Build history of the part. All positions in model axes, mm. A direction names the side the tool comes from. Give positions to 0.01 mm unless a question says otherwise; leave off trailing zeros. Write each loop counter-clockwise with the first axis right and the second up, starting at its lowest first coordinate (ties: lowest second). Pieces come first, ordered by that corner, then holes. Notation, with made-up numbers: M -1,50 L 44,50 A22 cw 44,70 Z; hole C 47.25,-26.75 d9. An arc over 180 degrees is marked long. One line per item, written item: value. Start each with the question number.
from build123d import *

# Parameters (mm, degrees)
SKETCH_1_R           = 1.6
EXTRUDE_1_DEPTH      = 2
SKETCH_2_R           = 12.5
CUT_EXTRUDE_1_DEPTH  = 3
SKETCH_5_R           = 26
SKETCH_5_R_2         = 22
EXTRUDE_3_DEPTH      = 10
EXTRUDE_5_DEPTH      = 10
SKETCH_15_R          = 1.65
CUT_EXTRUDE_2_DEPTH  = 42
SKETCH_16_R          = 1.65
CUT_EXTRUDE_3_DEPTH  = 42
CUT_EXTRUDE_4_DEPTH  = 18
CUT_EXTRUDE_5_DEPTH  = 18
EXTRUDE_6_DEPTH      = 45
SKETCH_24_W          = 50.26
SKETCH_24_H          = 14
EXTRUDE_7_DEPTH      = 5
SKETCH_25_R          = 1.65
CUT_EXTRUDE_6_DEPTH  = 5
CUT_EXTRUDE_7_DEPTH  = 3
CUT_EXTRUDE_9_DEPTH  = 10
CUT_EXTRUDE_START    = -8
CUT_EXTRUDE_10_DEPTH = 8
SKETCH_34_W          = 26
SKETCH_34_H          = 14
EXTRUDE_9_DEPTH      = 5
SKETCH_35_R          = 1.65
CUT_EXTRUDE_11_DEPTH = 5
CUT_EXTRUDE_12_DEPTH = 3
SKETCH_37_W          = 3
SKETCH_37_H          = 14
EXTRUDE_10_DEPTH     = 14


with BuildPart() as part:
    # 草图1 → 凸台-拉伸1 (new body)
    with BuildSketch(Plane(origin=(0, 0, 0), x_dir=(1, 0, 0), z_dir=(0, 1, 0))):
        with BuildLine():
            ThreePointArc((20.341082498, 8.380952381), (0, 22), (-20.341082498, 8.380952381))
            ThreePointArc((-20.341082498, 8.380952381), (-4.271778613, -21.581286048), (22, 0))
            ThreePointArc((22, 0), (21.581286048, 4.271778613), (20.341082498, 8.380952381))
        make_face()
        with Locations(Location((-12.727922061, -12.727922061, 0), (0, 0, 270))):
            Circle(SKETCH_1_R, mode=Mode.SUBTRACT)
        with Locations(Location((12.727922061, -12.727922061, 0), (0, 0, 270))):
            Circle(SKETCH_1_R, mode=Mode.SUBTRACT)
        with Locations(Location((-12.727922061, 12.727922061, 0), (0, 0, 270))):
            Circle(SKETCH_1_R, mode=Mode.SUBTRACT)
        with Locations(Location((12.727922061, 12.727922061, 0), (0, 0, 270))):
            Circle(SKETCH_1_R, mode=Mode.SUBTRACT)
    extrude(amount=EXTRUDE_1_DEPTH)

    # 草图2 → 切除-拉伸1 (cut)
    with BuildSketch(Plane(origin=(0, 2, 0), x_dir=(1, 0, 0), z_dir=(0, 1, 0))):
        with Locations(Location((0, 0, 0), (0, 0, 270))):
            Circle(SKETCH_2_R)
    extrude(amount=-CUT_EXTRUDE_1_DEPTH, mode=Mode.SUBTRACT)

    # 草图5 → 凸台-拉伸3 (add)
    with BuildSketch(Plane(origin=(0, 0, 0), x_dir=(1, 0, 0), z_dir=(0, 1, 0))):
        with Locations(Location((0, 0, 0), (0, 0, 270))):
            Circle(SKETCH_5_R)
        with Locations(Location((0, 0, 0), (0, 0, 270))):
            Circle(SKETCH_5_R_2, mode=Mode.SUBTRACT)
    extrude(amount=EXTRUDE_3_DEPTH)

    # 草图14 → 凸台-拉伸5 (add)
    with BuildSketch(Plane.XZ):
        with BuildLine():
            Line((-10.307764064, 20), (10.307764064, 20))
            ThreePointArc((10.307764064, 20), (15.909902577, 15.909902577), (20, 10.307764064))
            Line((20, 10.307764064), (20, -10.307764064))
            ThreePointArc((20, -10.307764064), (15.909902577, -15.909902577), (10.307764064, -20))
            Line((10.307764064, -20), (-10.307764064, -20))
            ThreePointArc((-10.307764064, -20), (-15.909902577, -15.909902577), (-20, -10.307764064))
            Line((-20, -10.307764064), (-20, 10.307764064))
            ThreePointArc((-20, 10.307764064), (-15.909902577, 15.909902577), (-10.307764064, 20))
        make_face()
        with BuildLine():
            Line((-9.013878189, 15), (9.013878189, 15))
            ThreePointArc((9.013878189, 15), (9.692559275, 14.570665555), (10.350828667, 14.110646544))
            ThreePointArc((10.350828667, 14.110646544), (14.67246571, 14.67246571), (14.110646544, 10.350828667))
            ThreePointArc((14.110646544, 10.350828667), (14.570665555, 9.692559275), (15, 9.013878189))
            Line((15, 9.013878189), (15, -9.013878189))
            ThreePointArc((15, -9.013878189), (14.570665555, -9.692559275), (14.110646544, -10.350828667))
            ThreePointArc((14.110646544, -10.350828667), (14.67246571, -14.67246571), (10.350828667, -14.110646544))
            ThreePointArc((10.350828667, -14.110646544), (9.692559275, -14.570665555), (9.013878189, -15))
            Line((9.013878189, -15), (-9.013878189, -15))
            ThreePointArc((-9.013878189, -15), (-9.692559275, -14.570665555), (-10.350828667, -14.110646544))
            ThreePointArc((-10.350828667, -14.110646544), (-14.67246571, -14.67246571), (-14.110646544, -10.350828667))
            ThreePointArc((-14.110646544, -10.350828667), (-14.570665555, -9.692559275), (-15, -9.013878189))
            Line((-15, -9.013878189), (-15, 9.013878189))
            ThreePointArc((-15, 9.013878189), (-14.570665555, 9.692559275), (-14.110646544, 10.350828667))
            ThreePointArc((-14.110646544, 10.350828667), (-14.67246571, 14.67246571), (-10.350828667, 14.110646544))
            ThreePointArc((-10.350828667, 14.110646544), (-9.692559275, 14.570665555), (-9.013878189, 15))
        make_face(mode=Mode.SUBTRACT)
    extrude(amount=EXTRUDE_5_DEPTH)

    # 草图15 → 切除-拉伸2 (cut)
    with BuildSketch(Plane.ZY.offset(20)):
        with Locations((0, -5)):
            Circle(SKETCH_15_R)
    extrude(amount=-CUT_EXTRUDE_2_DEPTH, mode=Mode.SUBTRACT)

    # 草图16 → 切除-拉伸3 (cut)
    with BuildSketch(Plane(origin=(0, 0, -20), x_dir=(-1, 0, 0), z_dir=(0, 0, -1))):
        with Locations((0, -5)):
            Circle(SKETCH_16_R)
    extrude(amount=-CUT_EXTRUDE_3_DEPTH, mode=Mode.SUBTRACT)

    # 草图18 → 切除-拉伸4 (cut, symmetric)
    with BuildSketch(Plane.XY):
        Polygon((-1.58771324, -2.25), (-3.175426481, -5), (-1.58771324, -7.75), (1.58771324, -7.75), (3.175426481, -5), (1.58771324, -2.25), align=None)
    extrude(amount=CUT_EXTRUDE_4_DEPTH, both=True, mode=Mode.SUBTRACT)

    # 草图19 → 切除-拉伸5 (cut, symmetric)
    with BuildSketch(Plane(origin=(0, 0, 0), x_dir=(0, 0, -1), z_dir=(1, 0, 0))):
        Polygon((-1.58771324, -2.25), (-3.175426481, -5), (-1.58771324, -7.75), (1.58771324, -7.75), (3.175426481, -5), (1.58771324, -2.25), align=None)
    extrude(amount=CUT_EXTRUDE_5_DEPTH, both=True, mode=Mode.SUBTRACT)

    # 草图23 → 凸台-拉伸6 (add)
    with BuildSketch(Plane(origin=(0, 10, 0), x_dir=(1, 0, 0), z_dir=(0, 1, 0))):
        with BuildLine():
            ThreePointArc((-22, 0), (-21.712282003, 3.546379878), (-20.856653615, 7))
            Line((-20.856653615, 7), (-25.039968051, 7))
            ThreePointArc((-25.039968051, 7), (-25.758873901, 3.53276313), (-26, 0))
            Line((-26, 0), (-22, 0))
        make_face()
        with BuildLine():
            ThreePointArc((-20.856653615, -7), (-21.712282003, -3.546379878), (-22, 0))
            Line((-22, 0), (-26, 0))
            ThreePointArc((-26, 0), (-25.758873901, -3.53276313), (-25.039968051, -7))
            Line((-25.039968051, -7), (-20.856653615, -7))
        make_face()
        with BuildLine():
            Line((25.039968051, 7), (20.856653615, 7))
            ThreePointArc((20.856653615, 7), (21.712282003, 3.546379878), (22, 0))
            Line((22, 0), (26, 0))
            ThreePointArc((26, 0), (25.758873901, 3.53276313), (25.039968051, 7))
        make_face()
        with BuildLine():
            Line((26, 0), (22, 0))
            ThreePointArc((22, 0), (21.712282003, -3.546379878), (20.856653615, -7))
            Line((20.856653615, -7), (25.039968051, -7))
            ThreePointArc((25.039968051, -7), (25.758873901, -3.53276313), (26, 0))
        make_face()
    extrude(amount=EXTRUDE_6_DEPTH)

    # 草图24 → 凸台-拉伸7 (add)
    with BuildSketch(Plane(origin=(0, 55, 0), x_dir=(1, 0, 0), z_dir=(0, 1, 0))):
        with Locations((-50.169968051, 0)):
            Rectangle(SKETCH_24_W, SKETCH_24_H)
    extrude_7 = extrude(amount=-EXTRUDE_7_DEPTH)

    # 镜向1: 凸台-拉伸7 across plane
    add(extrude_7.mirror(Plane(origin=(0, 0, 0), x_dir=(0, 0, 1), z_dir=(1, 0, 0))))

    # 草图25 → 切除-拉伸6 (cut)
    with BuildSketch(Plane(origin=(0, 55, 0), x_dir=(1, 0, 0), z_dir=(0, 1, 0))):
        with Locations(Location((-60.299968051, 0, 0), (0, 0, 270))):
            Circle(SKETCH_25_R)
        with Locations(Location((-30.299968051, 0, 0), (0, 0, 270))):
            Circle(SKETCH_25_R)
    cut_extrude_6 = extrude(amount=-CUT_EXTRUDE_6_DEPTH, mode=Mode.SUBTRACT)

    # 草图26 → 切除-拉伸7 (cut)
    with BuildSketch(Plane(origin=(0, 50, 0), x_dir=(1, 0, 0), z_dir=(0, 1, 0))):
        Polygon((-58.712254811, 2.75), (-61.887681291, 2.75), (-63.475394532, 0), (-61.887681291, -2.75), (-58.712254811, -2.75), (-57.124541571, 0), align=None)
        Polygon((-31.887681291, 2.75), (-33.475394532, 0), (-31.887681291, -2.75), (-28.712254811, -2.75), (-27.124541571, 0), (-28.712254811, 2.75), align=None)
    cut_extrude_7 = extrude(amount=CUT_EXTRUDE_7_DEPTH, mode=Mode.SUBTRACT)

    # 镜向3: 切除-拉伸6, 切除-拉伸7 across plane
    add(cut_extrude_6.mirror(Plane(origin=(0, 0, 0), x_dir=(0, 0, 1), z_dir=(1, 0, 0))), mode=Mode.SUBTRACT)
    add(cut_extrude_7.mirror(Plane(origin=(0, 0, 0), x_dir=(0, 0, 1), z_dir=(1, 0, 0))), mode=Mode.SUBTRACT)

    # 草图28 → 切除-拉伸9 (cut)
    with BuildSketch(Plane.XZ):
        with BuildLine():
            Line((-10.34, 20), (10.34, 20))
            Line((10.34, 20), (10.34, 23.855489934))
            ThreePointArc((10.34, 23.855489934), (0, 26), (-10.34, 23.855489934))
            Line((-10.34, 23.855489934), (-10.34, 20))
        make_face()
    extrude(amount=-CUT_EXTRUDE_9_DEPTH, mode=Mode.SUBTRACT)

    # 草图29 → 切除-拉伸10 (cut)
    with BuildSketch(Plane(origin=(0, 10, 0), x_dir=(1, 0, 0), z_dir=(0, 1, 0)).offset(CUT_EXTRUDE_START)):
        with BuildLine():
            Line((-10.34, -20), (-10.34, -19.418661128))
            ThreePointArc((-10.34, -19.418661128), (-9.756906344, -19.718082528), (-9.16515139, -20))
            Line((-9.16515139, -20), (-10.34, -20))
        make_face()
        with BuildLine():
            Line((10.34, -20), (10.34, -19.418661128))
            ThreePointArc((10.34, -19.418661128), (9.756906344, -19.718082528), (9.16515139, -20))
            Line((9.16515139, -20), (10.34, -20))
        make_face()
    extrude(amount=CUT_EXTRUDE_10_DEPTH, mode=Mode.SUBTRACT)

    # 草图34 → 凸台-拉伸9 (add)
    with BuildSketch(Plane.XZ.offset(-50)):
        with Locations((-88.299968051, 0)):
            Rectangle(SKETCH_34_W, SKETCH_34_H)
        with Locations((88.299968051, 0)):
            Rectangle(SKETCH_34_W, SKETCH_34_H)
    extrude(amount=-EXTRUDE_9_DEPTH)

    # 草图35 → 切除-拉伸11 (cut)
    with BuildSketch(Plane(origin=(0, 55, 0), x_dir=(1, 0, 0), z_dir=(0, 1, 0))):
        with Locations(Location((-90.299968051, 0, 0), (0, 0, 270))):
            Circle(SKETCH_35_R)
        with Locations(Location((90.299968051, 0, 0), (0, 0, 270))):
            Circle(SKETCH_35_R)
    extrude(amount=-CUT_EXTRUDE_11_DEPTH, mode=Mode.SUBTRACT)

    # 草图36 → 切除-拉伸12 (cut)
    with BuildSketch(Plane.XZ.offset(-50)):
        Polygon((-91.887681291, 2.75), (-93.475394532, 0), (-91.887681291, -2.75), (-88.712254811, -2.75), (-87.124541571, 0), (-88.712254811, 2.75), align=None)
        Polygon((91.887681291, 2.75), (88.712254811, 2.75), (87.124541571, 0), (88.712254811, -2.75), (91.887681291, -2.75), (93.475394532, 0), align=None)
    extrude(amount=-CUT_EXTRUDE_12_DEPTH, mode=Mode.SUBTRACT)

    # 草图37 → 凸台-拉伸10 (add)
    with BuildSketch(Plane.XZ.offset(-50)):
        with Locations((-102.799968051, 0)):
            Rectangle(SKETCH_37_W, SKETCH_37_H)
        with Locations((102.799968051, 0)):
            Rectangle(SKETCH_37_W, SKETCH_37_H)
    extrude(amount=-EXTRUDE_10_DEPTH)


solid = part.part
1) Probe line 1 along Y through (x, z) = (-19.6, 0); line 2 along X through (y, z) = (0.5, 0); line 3 along X through (y, z) = (-2, -8.5). List the from-to ranges inside material, lowest first. Write a range as from..to.
2) Drop flat-ended pins along their axis: P1, Ø15, axis at x = 0, z = 0, coming from the +Y side; P2, Ø16, axis at x = -57.5, y = 45, coming from the -Z side; P3, Ø2.5, axis at x = 0, z = 17, coming from the +Y side; P4, Ø1, axis at x = -17.5, z = 18, coming from the -Y side. Give the stop position or say it passes through.
3) Band-saw the part on B-B (x = -53.5). List the corners of the cut face in (y, z).
4) Tool access for faces 1 (the face through (-62, 55, 2)), 2 (the face through (-18, -6.2, -1.4)), 3 (the face through (-17, 10, 15)), 4 (the face through (92, 53, 1)): list every direction of +Z, -Z, +X, -X, +Y, -Y with a clear straight run to the whole face (end or side of a thin tool).
5) Band-saw the part on A-A (y = 35). List the corners of the cut face in (x, z), then the cut area to 3 significant figures.
6) Mould opens along X. For faces 5 (the face through (-14.622, -4.93, -14.722)), 6 (the face through (-15.98, -4.93, 15.84)), 7 (the face through (0, 0, -22)) say: released by +X, released by -X, zero draft, split by the parting line, or undercut.
Model answer:
1. line 1: y = -10..-6.65, -3.35..2
1. line 2: x = -26..-12.5, 12.5..26
1. line 3: x = -20..-15, 15..20
2. P1: passes through
2. P2: stops at z = -7
2. P3: stops at y = 2
2. P4: stops at y = 0
3. outline: M 50,-7 L 55,-7 L 55,7 L 50,7 Z
4. face 1: +Z, -Z, +Y
4. face 2: none
4. face 3: +Z, +X, -X, +Y
4. face 4: -Y
5. outline: M -25.04,-7 L -20.86,-7 A22 cw -20.86,7 L -25.04,7 A26 ccw Z; M 20.86,-7 L 25.04,-7 A26 ccw 25.04,7 L 20.86,7 A22 cw Z
5. area: 114 mm²
6. face 5: undercut
6. face 6: released by -X
6. face 7: zero draft
